CAD build for the part. Positions are in the model's coordinates, mm. Face numbers are marked on the shaded views. A direction names the side the tool comes from. Coordinates: 2 decimals unless noted, no trailing zeros. Loops run counter-clockwise (first coordinate to the right, second up) from the corner with the lowest first, then second, coordinate; pieces in that order, holes last. Notation, with made-up numbers: (53, -6.5) -> (87, -6.5) arc R31 ccw to (87, 30.5) -> close; hole circle Ø2 at (-30.75, 83.25). An arc over 180 degrees is marked (long way). Return JSON: item names as keys, results as strings. Group by question number.
(1) Tool access for the marked faces 1 and 2: list every direction of +Z, -Z, +X, -X, +Y, -Y with a clear straight run to the whole face (end or side of a thin tool).
(2) Flat gauge pins, fed straight in: pin 1 Ø1 at (y, z) = (2, 3) entering from -X; pin 2 Ø1.5 at (y, z) = (-5, 4.5) entering from -X; pin 3 Ø8 at (x, y) = (1, -12) entering from +Z. Where does each tip first touch, or does it go through?
(3) Mould opens along X. For the marked faces 3, 4, 5 and 6 say: pulls with the +X half, pulls with the -X half, needs draft (parallel to the pull), parting line crosses it, or undercut.
(4) Saw through at A-A on x = 0. Write the cut outline in (y, z).
(5) Saw through at B-B on y = -1.5. Write the cut outline in (x, z).
(6) Probe L1, parallel to Z at x = 0, y = -7; L2, parallel to X at y = -2.5, z = 0; L3, parallel to Y at x = 2, z = -12. List the from-to ranges inside material, lowest first.
```python
from build123d import *

# Parameters (mm, degrees)
CUT_EXTRUDE1_DEPTH = 43.728464961


with BuildPart() as part:
    # Sketch1 → Revolve1 (revolve)
    with BuildSketch(Plane.XY):
        with BuildLine():
            Line((0, -15.723376421), (0, 18.263376421))
            Line((0, 18.263376421), (17.041503786, 18.263376421))
            ThreePointArc((17.041503786, 18.263376421), (18.311503786, 16.993376421), (17.041503786, 15.723376421))
            Line((17.041503786, 15.723376421), (5.08, 15.723376421))
            Line((5.08, 15.723376421), (5.08, -15.723376421))
            Line((5.08, -15.723376421), (0, -15.723376421))
        make_face()
    revolve(axis=Axis((0, -15.723376421, 0), (0, 1, 0)))

    # Sketch2 → Cut-Extrude1 (cut, through all)
    with BuildSketch(Plane(origin=(0, 18.263376421, 0), x_dir=(1, 0, 0), z_dir=(0, 1, 0))):
        with BuildLine():
            Line((-0.604738857, -2.466959853), (-2.522366538, 0.298775913))
            ThreePointArc((-2.522366538, 0.298775913), (2.087347748, 1.447266174), (-0.604738857, -2.466959853))
        make_face()
    extrude(amount=-CUT_EXTRUDE1_DEPTH, mode=Mode.SUBTRACT)


solid = part.part
```
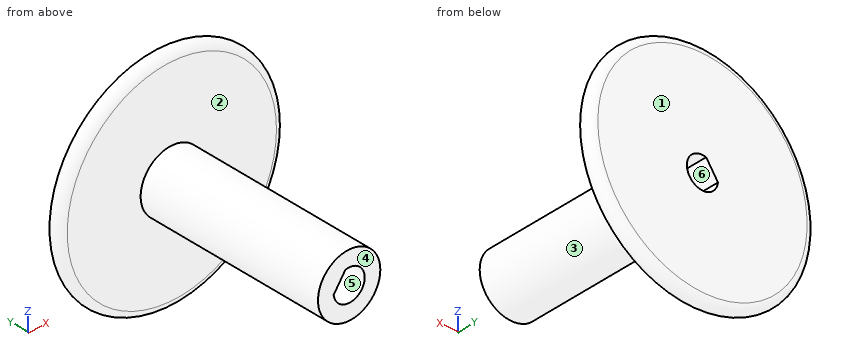
Geometry results:
{
 "1": {"face 1": "+Z, -Z, +X, -X, +Y", "face 2": "-Y"},
 "2": {"pin 1": "x = -4.42", "pin 2": "x = -3.43", "pin 3": "z = 5.08"},
 "3": {"face 3": "parting line crosses it", "face 4": "needs draft", "face 5": "undercut", "face 6": "undercut"},
 "4": {"outline": "(-15.72, -5.08) -> (15.72, -5.08) -> (15.72, -17.04) arc R1.27 ccw to (18.26, -17.04) -> (18.26, -2.54) -> (-15.72, -2.54) -> close; (-15.72, 2.54) -> (18.26, 2.54) -> (18.26, 17.04) arc R1.27 ccw to (15.72, 17.04) -> (15.72, 5.08) -> (-15.72, 5.08) -> close"},
 "5": {"outline": "circle Ø10.16 at (0, 0); hole (-2.52, -0.3) arc R2.54 ccw (long way) to (-0.6, 2.47) -> close"},
 "6": {"L1": "-5.08 to -2.54, 2.54 to 5.08", "L2": "-5.08 to -2.32, 2.54 to 5.08", "L3": "15.72 to 18.26"}
}
